Design review of the part built by this model. Coordinates are the model's own, in mm. Face numbers are marked on the shaded views. A direction names the side the tool comes from. Coordinates: 2 decimals unless noted, no trailing zeros. Write each loop counter-clockwise with the first axis right and the second up, starting at its lowest first coordinate (ties: lowest second). Pieces come first, ordered by that corner, then holes. Notation, with made-up numbers: (47, -16.5) - (72, -16.5) arc R11 cw to (72, 0.5) - close; hole circle Ø1 at (5.5, -40). An arc over 180 degrees is marked (long way). Answer as CSV lines item,"result". Start each with the question number.
Q1. Clearance check with flat-ended pins moving along their axes: pin 1 (1.2 mm diameter, centred on x = -1, y = 8, fed in from +Z); pin 2 (2 mm diameter, centred on x = -4, y = 8.5, fed in from -Z); pin 3 (0.6 mm diameter, centred on x = 26, y = 1.5, fed in from +Z). State where each tip first meets the part, or that it passes through.
Q2. Machinability: for the marked faces 4, 5, 6, 7 and 8, which of the approach directions +Z, -Z, +X, -X, +Y, -Y give a long, thin tool a straight path to every point of the face, cutting with its end or side? Answer none if there is none.
Q3. We need section A-A (x = 24). Write out the cut boundary in (y, z), plus the area to 3 significant figures.
Q4. For line 1 along Z through (x, y) = (24, 0.7); line 2 along Y through (x, z) = (6, -2); line 3 along Y through (x, z) = (-18, 3.5), list the stretches that pass through material, from the lowest coordinate up. Write a range as [from, to].
Q5. We need section C-C (x = -7). Write out the cut boundary in (y, z).
Q6. We need section D-D (y = 1.5). Write out the cut boundary in (x, z), plus the area to 3 significant figures.
Q7. Mouldability with a two-part tool opening along Y and no side actions: class the marked faces 1, 2 and 3 as pulls with the +Y half, pulls with the -Y half, needs draft (parallel to the pull), parting line crosses it, or undercut.
Q8. We need section B-B (y = -20.5). Write out the cut boundary in (x, z) (3 decimals), plus the area to 3 significant figures.
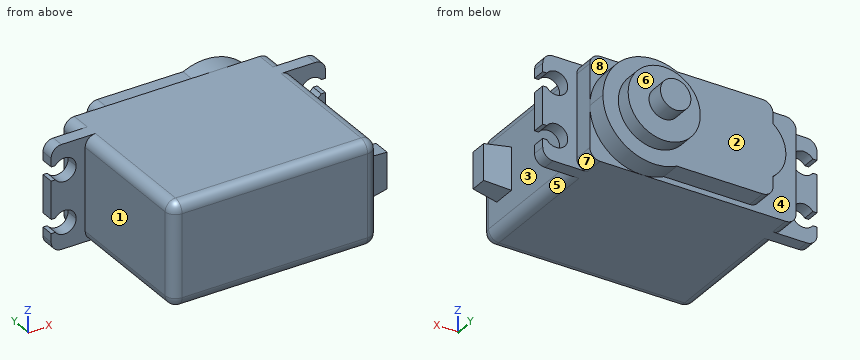
from build123d import *

# Parameters (mm, degrees)
BOSS_EXTRUDE1_DEPTH = 2.5
SKETCH2_W           = 40
SKETCH2_H           = 20
BOSS_EXTRUDE2_DEPTH = 4
SKETCH3_W           = 40
SKETCH3_H           = 20
BOSS_EXTRUDE3_DEPTH = 26.5
BOSS_EXTRUDE4_DEPTH = 4
SKETCH5_R           = 7
BOSS_EXTRUDE5_DEPTH = 3
SKETCH6_R           = 2.95
BOSS_EXTRUDE6_DEPTH = 3.5
FILLET1_R           = 2
SKETCH7_W           = 8.25
SKETCH7_H           = 4.5
BOSS_EXTRUDE7_DEPTH = 5
DRAFT3_ANGLE        = 7


with BuildPart() as part:
    # Sketch1 → Boss-Extrude1 (new body)
    with BuildSketch(Plane(origin=(0, 0, 0), x_dir=(1, 0, 0), z_dir=(0, 1, 0))):
        with BuildLine():
            ThreePointArc((25.8, 3.65), (21.75, 5), (25.8, 6.35))
            Line((25.8, 6.35), (26.6, 6.35))
            Line((26.6, 6.35), (26.6, 10))
            Line((26.6, 10), (-26.6, 10))
            Line((-26.6, 10), (-26.6, 6.35))
            Line((-26.6, 6.35), (-25.8, 6.35))
            ThreePointArc((-25.8, 6.35), (-23.288487526, 7.134537421), (-21.75, 5))
            ThreePointArc((-21.75, 5), (-23.288487526, 2.865462579), (-25.8, 3.65))
            Line((-25.8, 3.65), (-26.6, 3.65))
            Line((-26.6, 3.65), (-26.6, -3.65))
            Line((-26.6, -3.65), (-25.8, -3.65))
            ThreePointArc((-25.8, -3.65), (-23.288487526, -2.865462579), (-21.75, -5))
            ThreePointArc((-21.75, -5), (-23.288487526, -7.134537421), (-25.8, -6.35))
            Line((-25.8, -6.35), (-26.6, -6.35))
            Line((-26.6, -6.35), (-26.6, -10))
            Line((-26.6, -10), (26.6, -10))
            Line((26.6, -10), (26.6, -6.35))
            Line((26.6, -6.35), (25.8, -6.35))
            ThreePointArc((25.8, -6.35), (21.75, -5), (25.8, -3.65))
            Line((25.8, -3.65), (26.6, -3.65))
            Line((26.6, -3.65), (26.6, 3.65))
            Line((26.6, 3.65), (25.8, 3.65))
        make_face()
    extrude(amount=BOSS_EXTRUDE1_DEPTH)

    # Sketch2 → Boss-Extrude2 (add)
    with BuildSketch(Plane(origin=(0, 2.5, 0), x_dir=(1, 0, 0), z_dir=(0, 1, 0))):
        Rectangle(SKETCH2_W, SKETCH2_H)
    extrude(amount=BOSS_EXTRUDE2_DEPTH)

    # Sketch3 → Boss-Extrude3 (add)
    with BuildSketch(Plane.XZ):
        Rectangle(SKETCH3_W, SKETCH3_H)
    extrude(amount=BOSS_EXTRUDE3_DEPTH)

    # Sketch4 → Boss-Extrude4 (add)
    with BuildSketch(Plane(origin=(0, 6.5, 0), x_dir=(1, 0, 0), z_dir=(0, 1, 0))):
        with BuildLine():
            ThreePointArc((5.641101056, -9), (0, 0), (5.641101056, 9))
            Line((5.641101056, 9), (-13, 9))
            Line((-13, 9), (-13, 5))
            Line((-13, 5), (-13, -5))
            Line((-13, -5), (-13, -9))
            Line((-13, -9), (5.641101056, -9))
        make_face()
        with BuildLine():
            ThreePointArc((20, 0), (15.310885546, 8.473163206), (5.641101056, 9))
            Line((5.641101056, 9), (5.641101056, -9))
            ThreePointArc((5.641101056, -9), (15.310885546, -8.473163206), (20, 0))
        make_face()
        with BuildLine():
            Line((5.641101056, -9), (5.641101056, 9))
            ThreePointArc((5.641101056, 9), (0, 0), (5.641101056, -9))
        make_face()
        with BuildLine():
            Line((-13, -5), (-13, 5))
            ThreePointArc((-13, 5), (-15.5, 0), (-13, -5))
        make_face()
    extrude(amount=BOSS_EXTRUDE4_DEPTH)

    # Sketch5 → Boss-Extrude5 (add)
    with BuildSketch(Plane(origin=(0, 10.5, 0), x_dir=(1, 0, 0), z_dir=(0, 1, 0))):
        with Locations((10, 0)):
            Circle(SKETCH5_R)
    extrude(amount=BOSS_EXTRUDE5_DEPTH)

    # Sketch6 → Boss-Extrude6 (add)
    with BuildSketch(Plane(origin=(0, 13.5, 0), x_dir=(1, 0, 0), z_dir=(0, 1, 0))):
        with Locations((10, 0)):
            Circle(SKETCH6_R)
    extrude(amount=BOSS_EXTRUDE6_DEPTH)

    # Fillet1
    fillet1_edges = [part.edges().sort_by_distance(p)[0] for p in [
        (-26.6, 1.25, -10),
        (26.6, 1.25, -10),
        (26.6, 1.25, 10),
        (-26.6, 1.25, 10),
        (-20, 4.5, -10),
        (-20, 4.5, 10),
        (20, 4.5, 10),
        (20, 4.5, -10),
        (20, -13.25, 10),
        (-20, -26.5, 0),
        (-20, -13.25, 10),
        (0, -26.5, -10),
        (-20, -13.25, -10),
        (20, -13.25, -10),
        (0, -26.5, 10),
        (20, -26.5, 0),
        (-13, 8.5, 9),
        (-13, 8.5, -9),
    ]]
    fillet(fillet1_edges, radius=FILLET1_R)

    # Sketch7 → Boss-Extrude7 (add)
    with BuildSketch(Plane(origin=(20, 0, 0), x_dir=(0, 0, -1), z_dir=(1, 0, 0))):
        with Locations((0, -19.75000011)):
            Rectangle(SKETCH7_W, SKETCH7_H)
    extrude(amount=BOSS_EXTRUDE7_DEPTH)

    # Draft3
    draft3_faces = [part.faces().sort_by_distance(p)[0] for p in [
        (22.5, -22.00000011, 0),
        (22.5, -19.75000011, 4.125),
        (22.5, -19.75000011, -4.125),
        (22.5, -17.50000011, 0),
    ]]
    draft(draft3_faces, Plane(origin=(20, -26.5, -10), x_dir=(0, 0, 1), z_dir=(1, 0, 0)), DRAFT3_ANGLE)


solid = part.part
Results list:
1,pin 1,"stops at z = 9"
1,pin 2,"stops at z = -9"
1,pin 3,"stops at z = 9.67"
2,face 4,"-X, +Y"
2,face 5,"-Z, +X, -Y"
2,face 6,"+Y"
2,face 7,"-Z, +X, +Y"
2,face 8,"+Z, +X, +Y"
3,outline,"(-21.51, -3.63) - (-17.99, -3.63) - (-17.99, 3.63) - (-21.51, 3.63) - close; (0, -10) - (2.5, -10) - (2.5, -7.25) - (0, -7.25) - close; (0, -2.75) - (2.5, -2.75) - (2.5, 2.75) - (0, 2.75) - close; (0, 7.25) - (2.5, 7.25) - (2.5, 10) - (0, 10) - close"
3,area,"53.1 mm2"
4,line 1,"z = [-10, -7.25], [-2.75, 2.75], [7.25, 10]"
4,line 2,"y = [-26.5, 13.5]"
4,line 3,"y = [-26.5, 6.5]"
5,outline,"(-26.5, -8) arc R2 ccw to (-24.5, -10) - (6.5, -10) - (6.5, -9) - (10.5, -9) - (10.5, 9) - (6.5, 9) - (6.5, 10) - (-24.5, 10) arc R2 ccw to (-26.5, 8) - close"
6,outline,"(-26.6, -8) arc R2 ccw to (-24.6, -10) - (24.6, -10) arc R2 ccw to (26.6, -8) - (26.6, -6.35) - (25.8, -6.35) arc R2.25 cw (long way) to (25.8, -3.65) - (26.6, -3.65) - (26.6, 3.65) - (25.8, 3.65) arc R2.25 cw (long way) to (25.8, 6.35) - (26.6, 6.35) - (26.6, 8) arc R2 ccw to (24.6, 10) - (-24.6, 10) arc R2 ccw to (-26.6, 8) - (-26.6, 6.35) - (-25.8, 6.35) arc R2.25 cw (long way) to (-25.8, 3.65) - (-26.6, 3.65) - (-26.6, -3.65) - (-25.8, -3.65) arc R2.25 cw (long way) to (-25.8, -6.35) - (-26.6, -6.35) - close"
6,area,"992 mm2"
7,face 1,"needs draft"
7,face 2,"pulls with the +Y half"
7,face 3,"undercut"
8,outline,"(-20, -8) arc R2 ccw to (-18, -10) - (18, -10) arc R2 ccw to (20, -8) - (20, -4.125) - (25, -3.511) - (25, 3.511) - (20, 4.125) - (20, 8) arc R2 ccw to (18, 10) - (-18, 10) arc R2 ccw to (-20, 8) - close"
8,area,"835 mm2"
